Answer from the drawing. Dimensions are ordinates in mm from the lowest x, y and z of the part. Coordinates: 2 decimals unless noted, no trailing zeros. Loops run counter-clockwise (first coordinate to the right, second up) from the corner with the lowest first, then second, coordinate; pieces in that order, holes last. Notation, with made-up numbers: M 25,32.25 L 73,32.25 A4 ccw 73,36.25 Z; hole C 39.5,19.25 d6. An arc over 180 degrees is marked long. Put each result on its own line as item: value.
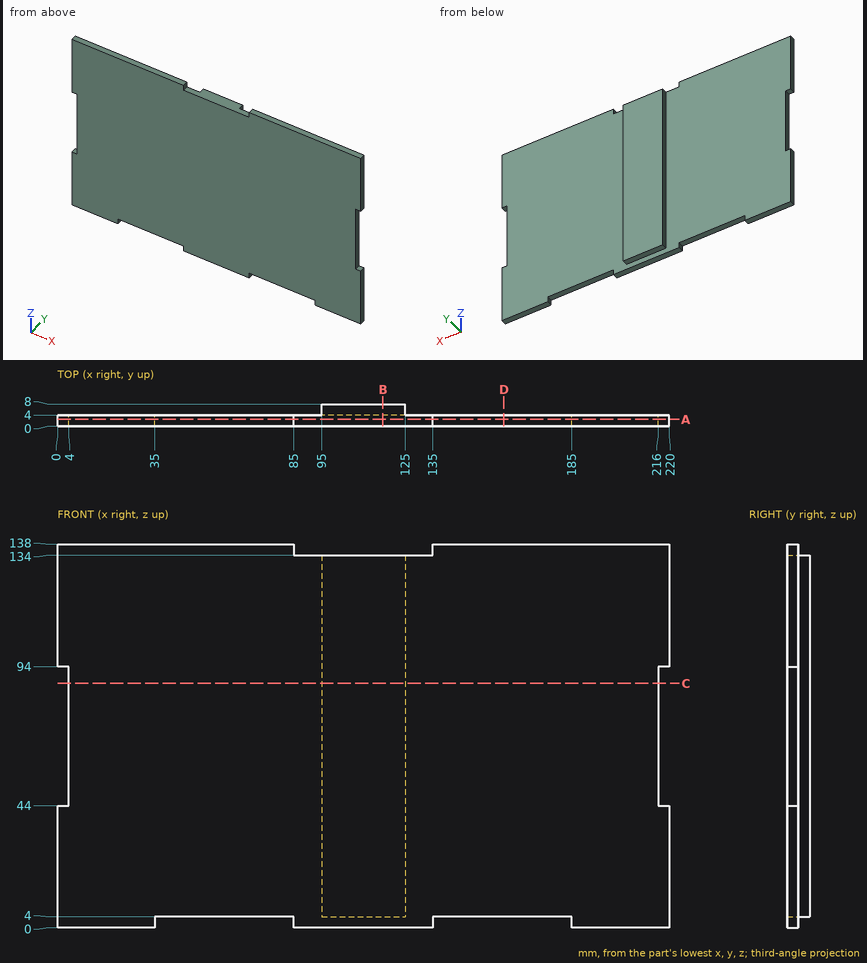
1) Find section A-A, the plane y = 2.5. Write down the section's boundary in (x, z), plus the area to 3 significant figures.
Answer list:
outline: M 0,0 L 35,0 L 35,4 L 85,4 L 85,0 L 135,0 L 135,4 L 185,4 L 185,0 L 220,0 L 220,44 L 216,44 L 216,94 L 220,94 L 220,138 L 135,138 L 135,134 L 85,134 L 85,138 L 0,138 L 0,94 L 4,94 L 4,44 L 0,44 Z
area: 29,400 mm^2
2) Find section D-D, the plane x = 160.5. Write down the section's boundary in (y, z).
Answer list:
outline: M 0,4 L 4,4 L 4,138 L 0,138 Z
3) Given pin 1 Ø2 at (y, z) = (4, 56.5) entering from -X; pin 2 Ø3 at (y, z) = (2, 73.5) entering from +X; pin 3 Ø12 at (x, z) = (56, 25.5) entering from +Y, each flat-ended and moving along its own axis, determine where each tip first touches the part or whether it passes through.
Answer list:
pin 1: stops at x = 4
pin 2: stops at x = 216
pin 3: stops at y = 4
4) Find section C-C, the plane z = 88. Write down the section's boundary in (x, y).
Answer list:
outline: M 4,0 L 216,0 L 216,4 L 125,4 L 125,8 L 95,8 L 95,4 L 4,4 Z
5) Find section B-B, the plane x = 117. Write down the section's boundary in (y, z), plus the area to 3 significant figures.
Answer list:
outline: M 0,0 L 4,0 L 4,4 L 8,4 L 8,134 L 0,134 Z
area: 1,060 mm^2
6) Straight lines are drawn through the part: line 1 (X direction, y = 4.75, z = 74); line 2 (Y direction, x = 22.5, z = 96); line 3 (Z direction, x = 86, y = 0.5). For each, find the intervals that lie inside material, in ascending order. Write a range as [from, to].
Answer list:
line 1: x = [95, 125]
line 2: y = [0, 4]
line 3: z = [0, 134]
